```python
from build123d import *

# Parameters (mm, degrees)
SKETCH1_W           = 275
SKETCH1_H           = 145.5
BOSS_EXTRUDE1_DEPTH = 102.5
SKETCH3_W           = 115
SKETCH3_H           = 45.5
SKETCH3_W_2         = 80
SKETCH3_H_2         = 40
CUT_EXTRUDE1_DEPTH  = 102.5
SKETCH4_W           = 80
SKETCH4_H           = 82.5
CUT_EXTRUDE3_DEPTH  = 100
CUT_EXTRUDE4_DEPTH  = 105.5
SKETCH7_W           = 20
SKETCH7_H           = 31.25
SKETCH7_H_2         = 31.588652779
CUT_EXTRUDE5_DEPTH  = 105.5
CUT_EXTRUDE7_DEPTH  = 85.5
SKETCH10_W          = 100
SKETCH10_H          = 48.75
CUT_EXTRUDE8_DEPTH  = 14
SKETCH11_W          = 100
SKETCH11_H          = 48.75
CUT_EXTRUDE9_DEPTH  = 14
SKETCH12_W          = 10
SKETCH12_H          = 48.75
CUT_EXTRUDE10_DEPTH = 26
SKETCH13_W          = 10
SKETCH13_H          = 48.75
CUT_EXTRUDE12_DEPTH = 26
SKETCH14_W          = 15
SKETCH14_H          = 48.75
CUT_EXTRUDE13_DEPTH = 80
CUT_EXTRUDE14_DEPTH = 102.5
CUT_EXTRUDE15_DEPTH = 48.75
CUT_EXTRUDE16_DEPTH = 48.75
CUT_EXTRUDE17_DEPTH = 5
CUT_EXTRUDE18_DEPTH = 105
SKETCH24_R          = 5
CUT_EXTRUDE19_DEPTH = 105
CUT_EXTRUDE20_DEPTH = 105
FILLET1_R           = 10
FILLET2_R           = 10
FILLET3_R           = 10
FILLET4_R           = 10
FILLET5_R           = 10
FILLET6_R           = 10
FILLET7_R           = 10
FILLET8_R           = 10
FILLET9_R           = 10
FILLET10_R          = 10
FILLET11_R          = 10
FILLET12_R          = 10


with BuildPart() as part:
    # Sketch1 → Boss-Extrude1 (new body)
    with BuildSketch(Plane.XY):
        with Locations((93.302092116, 48.653058441)):
            Rectangle(SKETCH1_W, SKETCH1_H)
    extrude(amount=BOSS_EXTRUDE1_DEPTH)

    # Sketch3 → Cut-Extrude1 (cut)
    with BuildSketch(Plane.XY.offset(102.5)):
        with Locations((13.302092116, 98.653058441)):
            Rectangle(SKETCH3_W, SKETCH3_H)
        with Locations((190.802092116, -4.096941559)):
            Rectangle(SKETCH3_W_2, SKETCH3_H_2)
    extrude(amount=-CUT_EXTRUDE1_DEPTH, mode=Mode.SUBTRACT)

    # Sketch4 → Cut-Extrude3 (cut)
    with BuildSketch(Plane(origin=(0, 75.903058441, 0), x_dir=(1, 0, 0), z_dir=(0, 1, 0))):
        with Locations((5.802092116, -51.25)):
            Rectangle(SKETCH4_W, SKETCH4_H)
    extrude(amount=-CUT_EXTRUDE3_DEPTH, mode=Mode.SUBTRACT)

    # Sketch6 → Cut-Extrude4 (cut)
    with BuildSketch(Plane(origin=(0, 121.403058441, 0), x_dir=(1, 0, 0), z_dir=(0, 1, 0))):
        Polygon((200.803509438, -51.25), (200.803509438, -41.25), (220.802092116, -41.25), (220.802092116, -51.25), (220.802092116, -61.25), (200.803509438, -61.25), align=None)
    extrude(amount=-CUT_EXTRUDE4_DEPTH, mode=Mode.SUBTRACT)

    # Sketch7 → Cut-Extrude5 (cut)
    with BuildSketch(Plane(origin=(0, 121.403058441, 0), x_dir=(1, 0, 0), z_dir=(0, 1, 0))):
        with Locations((220.802092116, -15.625)):
            Rectangle(SKETCH7_W, SKETCH7_H)
        with Locations((220.802092116, -87.04432639)):
            Rectangle(SKETCH7_W, SKETCH7_H_2)
    extrude(amount=-CUT_EXTRUDE5_DEPTH, mode=Mode.SUBTRACT)

    # Sketch8 → Cut-Extrude7 (cut)
    with BuildSketch(Plane(origin=(0, 121.403058441, 0), x_dir=(1, 0, 0), z_dir=(0, 1, 0))):
        Polygon((190.802092116, -31.25), (190.802092116, -48.75), (70.802092116, -48.75), (70.802092116, 0), (210.802092116, 0), (210.802092116, -31.25), align=None)
        Polygon((190.802092116, -71.25), (190.802092116, -53.75), (70.802092116, -53.75), (70.802092116, -102.5), (210.802092116, -102.5), (210.802092116, -71.25), align=None)
    extrude(amount=-CUT_EXTRUDE7_DEPTH, mode=Mode.SUBTRACT)

    # Sketch10 → Cut-Extrude8 (cut)
    with BuildSketch(Plane(origin=(0, 35.903058441, 0), x_dir=(1, 0, 0), z_dir=(0, 1, 0))):
        with Locations((120.802092116, -78.125)):
            Rectangle(SKETCH10_W, SKETCH10_H)
    extrude(amount=-CUT_EXTRUDE8_DEPTH, mode=Mode.SUBTRACT)

    # Sketch11 → Cut-Extrude9 (cut)
    with BuildSketch(Plane(origin=(0, 35.903058441, 0), x_dir=(1, 0, 0), z_dir=(0, 1, 0))):
        with Locations((120.802092116, -24.375)):
            Rectangle(SKETCH11_W, SKETCH11_H)
    extrude(amount=-CUT_EXTRUDE9_DEPTH, mode=Mode.SUBTRACT)

    # Sketch12 → Cut-Extrude10 (cut)
    with BuildSketch(Plane(origin=(0, 21.903058441, 0), x_dir=(1, 0, 0), z_dir=(0, 1, 0))):
        with Locations((75.802092116, -78.125)):
            Rectangle(SKETCH12_W, SKETCH12_H)
    extrude(amount=-CUT_EXTRUDE10_DEPTH, mode=Mode.SUBTRACT)

    # Sketch13 → Cut-Extrude12 (cut)
    with BuildSketch(Plane(origin=(0, 21.903058441, 0), x_dir=(1, 0, 0), z_dir=(0, 1, 0))):
        with Locations((75.802092116, -24.375)):
            Rectangle(SKETCH13_W, SKETCH13_H)
    extrude(amount=-CUT_EXTRUDE12_DEPTH, mode=Mode.SUBTRACT)

    # Sketch14 → Cut-Extrude13 (cut)
    with BuildSketch(Plane(origin=(0, 75.903058441, 0), x_dir=(1, 0, 0), z_dir=(0, 1, 0))):
        with Locations((63.302092116, -78.125)):
            Rectangle(SKETCH14_W, SKETCH14_H)
        with Locations((63.302092116, -24.375)):
            Rectangle(SKETCH14_W, SKETCH14_H)
    extrude(amount=-CUT_EXTRUDE13_DEPTH, mode=Mode.SUBTRACT)

    # Sketch16 → Cut-Extrude14 (cut)
    with BuildSketch(Plane.XY.offset(102.5)):
        Polygon((150.802092116, 15.903058441), (117.238106869, -24.096941559), (150.802092116, -24.096941559), align=None)
    extrude(amount=-CUT_EXTRUDE14_DEPTH, mode=Mode.SUBTRACT)

    # Sketch17 → Cut-Extrude15 (cut)
    with BuildSketch(Plane.XY.offset(102.5)):
        Polygon((80.802092116, -4.096941559), (80.802092116, -18.096941559), (114.44026092, -18.096941559), (148.004246167, 21.903058441), (80.802092116, 21.903058441), align=None)
    extrude(amount=-CUT_EXTRUDE15_DEPTH, mode=Mode.SUBTRACT)

    # Sketch18 → Cut-Extrude16 (cut)
    with BuildSketch(Plane(origin=(0, 0, 0), x_dir=(-1, 0, 0), z_dir=(0, 0, -1))):
        Polygon((-80.802092116, -4.096941559), (-80.802092116, -18.096941559), (-114.44026092, -18.096941559), (-148.004246167, 21.903058441), (-80.802092116, 21.903058441), align=None)
    extrude(amount=-CUT_EXTRUDE16_DEPTH, mode=Mode.SUBTRACT)

    # Sketch19 → Cut-Extrude17 (cut)
    with BuildSketch(Plane.XY.offset(53.75)):
        Polygon((70.802092116, 75.903058441), (134.245946408, 75.903058441), (172.424979627, 121.403058441), (70.802092116, 121.403058441), align=None)
    extrude(amount=-CUT_EXTRUDE17_DEPTH, mode=Mode.SUBTRACT)

    # Sketch23 → Cut-Extrude18 (cut)
    with BuildSketch(Plane.XZ.offset(24.096941559)):
        Polygon((11.802092116, 102.5), (210.802092116, 71.25), (210.802092116, 102.5), align=None)
    extrude(amount=-CUT_EXTRUDE18_DEPTH, mode=Mode.SUBTRACT)

    # Sketch24 → Cut-Extrude19 (cut)
    with BuildSketch(Plane(origin=(0, 0, 0), x_dir=(-1, 0, 0), z_dir=(0, 0, -1))):
        with Locations((-180.802092116, 25.903058441)):
            Circle(SKETCH24_R)
        with Locations((-70.802092116, -14.096941559)):
            Circle(SKETCH24_R)
    extrude(amount=-CUT_EXTRUDE19_DEPTH, mode=Mode.SUBTRACT)

    # Sketch25 → Cut-Extrude20 (cut)
    with BuildSketch(Plane.XZ.offset(24.096941559)):
        Polygon((11.802092116, 0), (210.802092116, 0), (210.802092116, 31.25), align=None)
    extrude(amount=-CUT_EXTRUDE20_DEPTH, mode=Mode.SUBTRACT)

    # Fillet1
    fillet1_edges = [part.edges().sort_by_distance(p)[0] for p in [
        (80.802092116, -4.096941559, 72.707286432),
    ]]
    fillet(fillet1_edges, radius=FILLET1_R)

    # Fillet2
    fillet2_edges = [part.edges().sort_by_distance(p)[0] for p in [
        (148.004246167, 21.903058441, 67.430735392),
    ]]
    fillet(fillet2_edges, radius=FILLET2_R)

    # Fillet3
    fillet3_edges = [part.edges().sort_by_distance(p)[0] for p in [
        (170.802092116, 35.903058441, 65.640703518),
    ]]
    fillet(fillet3_edges, radius=FILLET3_R)

    # Fillet4
    fillet4_edges = [part.edges().sort_by_distance(p)[0] for p in [
        (80.802092116, -4.096941559, 29.792713568),
    ]]
    fillet(fillet4_edges, radius=FILLET4_R)

    # Fillet5
    fillet5_edges = [part.edges().sort_by_distance(p)[0] for p in [
        (148.004246167, 21.903058441, 35.069264608),
    ]]
    fillet(fillet5_edges, radius=FILLET5_R)

    # Fillet6
    fillet6_edges = [part.edges().sort_by_distance(p)[0] for p in [
        (170.802092116, 35.903058441, 36.859296482),
    ]]
    fillet(fillet6_edges, radius=FILLET6_R)

    # Fillet7
    fillet7_edges = [part.edges().sort_by_distance(p)[0] for p in [
        (114.44026092, -18.096941559, 32.433901445),
    ]]
    fillet(fillet7_edges, radius=FILLET7_R)

    # Fillet8
    fillet8_edges = [part.edges().sort_by_distance(p)[0] for p in [
        (114.44026092, -18.096941559, 70.066098555),
    ]]
    fillet(fillet8_edges, radius=FILLET8_R)

    # Fillet9
    fillet9_edges = [part.edges().sort_by_distance(p)[0] for p in [
        (134.245946408, 75.903058441, 51.25),
    ]]
    fillet(fillet9_edges, radius=FILLET9_R)

    # Fillet10
    fillet10_edges = [part.edges().sort_by_distance(p)[0] for p in [
        (172.424979627, 121.403058441, 51.25),
    ]]
    fillet(fillet10_edges, radius=FILLET10_R)

    # Fillet11
    fillet11_edges = [part.edges().sort_by_distance(p)[0] for p in [
        (150.802092116, 15.903058441, 51.25),
    ]]
    fillet(fillet11_edges, radius=FILLET11_R)

    # Fillet12
    fillet12_edges = [part.edges().sort_by_distance(p)[0] for p in [
        (117.238106869, -24.096941559, 51.25),
    ]]
    fillet(fillet12_edges, radius=FILLET12_R)


solid = part.part
```
CAD build for the part. Positions are in the model's coordinates, mm. A direction names the side the tool comes from. Round coordinates to 2 decimals unless told otherwise and drop trailing zeros. Write each loop counter-clockwise with the first axis right and the second up, starting at its lowest first coordinate (ties: lowest second). Pieces come first, ordered by that corner, then holes. Notation, with made-up numbers: (26, 78) -> (40, 78) arc R26 ccw to (40, 108) -> close; hole circle Ø4 at (-27, 56). An arc over 180 degrees is marked (long way). Answer in a Markdown table with one row per item. Add a question column.
Item 1: Which spindle directions (+Z, -Z, +X, -X, +Y, -Y) get a long thin tool onto all of the face, cutting with end or side? Do faces 4 (the face through (49, 75.903, 55)), 5 (the face through (190.802, 79, 63)), 6 (the face through (95, -18.097, 30)). Say none if no direction does.
Item 2: Mould opens along X. For faces 1 (the face through (51.875, 18.262, 96.207)), 2 (the face through (-17, 27, 102.5)), 3 (the face through (122, 53, 53.75)) say: pulls with the +X half, pulls with the -X half, needs draft (parallel to the pull), parting line crosses it, or undercut.
Item 3: Saw through at A-A, the plane z = 67. Write the cut outline in (x, y).
Item 4: Saw through at C-C, the plane y = 63. Write the cut outline in (x, z).
Item 5: Drill centre lines: line 1 (X direction, y = 68, z = 54); line 2 (X direction, y = 9, z = 24); line 3 (X direction, y = 43, z = 65.5). Where is each one in solid material? Low to high. Write a range as from..to.
Item 6: Saw through at D-D, the plane y = 103. Write the cut outline in (x, z), then the cut area to 3 significant figures.
Item 7: Drop flat-ended pins along their axis: pin 1 Ø2 at (x, y) = (153.5, 27) entering from -Z; pin 2 Ø14.5 at (x, z) = (158.5, 35.5) entering from +Y; pin 3 Ø4 at (x, z) = (55, 46) entering from +Y. Give the stop position or say it passes through.
Item 8: Saw through at B-B, the plane x = 214.5. Write the cut outline in (y, z), then the cut area to 3 significant figures.
Findings below:
| question | item | result |
|---|---|---|
| 1 | face 4 | +Z, -Z, -X, +Y |
| 1 | face 5 | +Z, +Y |
| 1 | face 6 | -Z, +Y |
| 2 | face 1 | pulls with the +X half |
| 2 | face 2 | needs draft |
| 2 | face 3 | undercut |
| 3 | outline | (-44.2, -24.1) -> (-34.2, -24.1) -> (-34.2, 75.9) -> (-44.2, 75.9) -> close; (45.8, -24.1) -> (112.58, -24.1) arc R10 ccw to (120.24, -20.52) -> (147.8, 12.33) arc R10 cw to (155.47, 15.9) -> (230.8, 15.9) -> (230.8, 121.4) -> (190.8, 121.4) -> (190.8, 35.9) -> (180.8, 35.9) arc R10 ccw to (170.8, 25.9) -> (170.8, 21.9) -> (152.67, 21.9) arc R10 ccw to (145.01, 18.33) -> (117.44, -14.52) arc R10 cw to (109.78, -18.1) -> (80.8, -18.1) -> (80.8, -14.1) arc R10 ccw to (70.8, -4.1) -> (55.8, -4.1) -> (55.8, 75.9) -> (45.8, 75.9) -> close; hole circle Ø10 at (70.8, -14.1); hole circle Ø10 at (180.8, 25.9) |
| 4 | outline | (-44.2, 0) -> (11.8, 0) -> (55.8, 6.91) -> (55.8, 48.75) -> (190.8, 48.75) -> (190.8, 31.25) -> (230.8, 31.25) -> (230.8, 71.25) -> (190.8, 71.25) -> (190.8, 53.75) -> (55.8, 53.75) -> (55.8, 95.59) -> (11.8, 102.5) -> (-44.2, 102.5) -> close; hole (-34.2, 10) -> (45.8, 10) -> (45.8, 92.5) -> (-34.2, 92.5) -> close; hole (200.8, 41.25) -> (220.8, 41.25) -> (220.8, 61.25) -> (200.8, 61.25) -> close |
| 5 | line 1 | x = -44.2..-34.2, 45.8..55.8, 190.8..200.8, 220.8..230.8 |
| 5 | line 2 | x = -44.2..-34.2, 45.8..55.8, 137.18..145.01 |
| 5 | line 3 | x = -44.2..-34.2, 45.8..55.8, 190.8..230.8 |
| 6 | outline | (156.98, 48.75) -> (190.8, 48.75) -> (190.8, 31.25) -> (230.8, 31.25) -> (230.8, 71.25) -> (190.8, 71.25) -> (190.8, 53.75) -> (156.98, 53.75) -> close; hole (200.8, 41.25) -> (220.8, 41.25) -> (220.8, 61.25) -> (200.8, 61.25) -> close |
| 6 | area | 1,370 mm^2 |
| 7 | pin 1 | stops at z = 48.75 |
| 7 | pin 2 | stops at y = 21.9 |
| 7 | pin 3 | stops at y = 75.9 |
| 8 | outline | (15.9, 31.25) -> (121.4, 31.25) -> (121.4, 41.25) -> (15.9, 41.25) -> close; (15.9, 61.25) -> (121.4, 61.25) -> (121.4, 71.25) -> (15.9, 71.25) -> close |
| 8 | area | 2,110 mm^2 |
